from build123d import *

# Parameters (mm, degrees)
F1_DEPTH = 19.05


with BuildPart() as f1:
    # F0 (on Top) → F1 (new body)
    with BuildSketch(Plane.XY):
        with BuildLine():
            ThreePointArc((-100.25353, 101.826), (-101.667744, 101.240213), (-102.25353, 99.826))
            Line((-102.25353, 99.826), (-102.25353, -10.474))
            ThreePointArc((-102.25353, -10.474), (-101.667744, -11.888214), (-100.25353, -12.474))
            Line((-100.25353, -12.474), (-10.564581, -12.474))
            ThreePointArc((-10.564581, -12.474), (-10.036438, -12.544994), (-9.545789, -12.752936))
            Line((-9.545789, -12.752936), (77.88431, -64.507527))
            ThreePointArc((77.88431, -64.507527), (79.399684, -64.723833), (80.624166, -63.805253))
            Line((80.624166, -63.805253), (117.402527, -1.674808))
            ThreePointArc((117.402527, -1.674808), (117.618833, -0.159434), (116.700253, 1.065048))
            Line((116.700253, 1.065048), (51.127679, 39.880991))
            ThreePointArc((51.127679, 39.880991), (50.409003, 40.611496), (50.14647, 41.602056))
            Line((50.14647, 41.602056), (50.14647, 87.126))
            ThreePointArc((50.14647, 87.126), (49.560684, 88.540213), (48.14647, 89.126))
            Line((48.14647, 89.126), (-28.05353, 89.126))
            ThreePointArc((-28.05353, 89.126), (-28.549656, 89.188512), (-29.014768, 89.37214))
            Line((-29.014768, 89.37214), (-51.28878, 101.579859))
            ThreePointArc((-51.28878, 101.579859), (-51.753892, 101.763487), (-52.250017, 101.826))
            Line((-52.250017, 101.826), (-100.25353, 101.826))
        make_face()
    extrude(amount=F1_DEPTH)


solid = f1.part
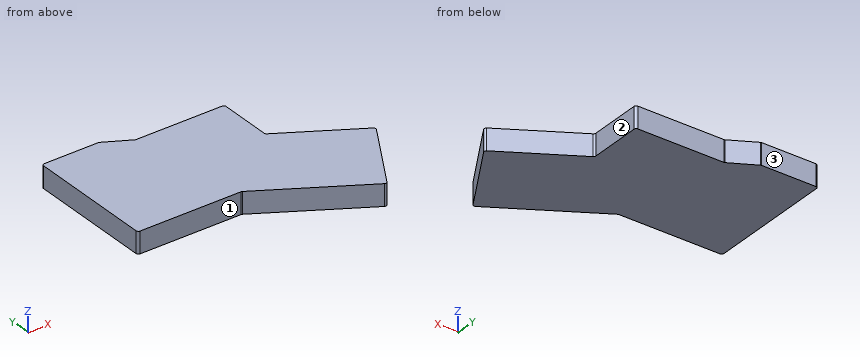
Can you work these out from the model? Positions are in its coordinate system, mm. Face numbers are marked on the shaded views. A direction names the side the tool comes from. Coordinates: 2 decimals unless noted, no trailing zeros. Write each loop counter-clockwise with the first axis right and the second up, starting at its lowest first coordinate (ties: lowest second). Pieces come first, ordered by that corner, then holes. Notation, with made-up numbers: M 17,0 L 75,0 A5 ccw 75,5 Z; hole C -28.5,22.25 d5. An arc over 180 degrees is marked long. Use one line per item in the form item = value.
Q1. I need wall thicknesses on line 1 along Y through (x, z) = (-90, 8.5); line 2 along Y through (x, z) = (-15, 10.5); line 3 along X through (y, z) = (68, 14). Which ranges of each line are inside material? Lowest first, please. Write a range as from..to.
Model answer:
line_1 = -12.47..101.83
line_2 = -12.47..89.13
line_3 = -102.25..50.15
Q2. For the marked faces 1, 2 and 3, which set-ups out of +Z, -Z, +X, -X, +Y, -Y let a thin tool reach every point of the face, with its end or its side?
Model answer:
face_1 = +Z, -Z, -X, -Y
face_2 = +Z, -Z, +X, +Y
face_3 = +Z, -Z, +X, -X, +Y
Q3. If we section it at B-B (x = -88.5): Write out the boundary of the cut face in (y, z).
Model answer:
outline = M -12.47,0 L 101.83,0 L 101.83,19.05 L -12.47,19.05 Z
Q4. If we section it at C-C (y = 73): Write out the boundary of the cut face in (x, z).
Model answer:
outline = M -102.25,0 L 50.15,0 L 50.15,19.05 L -102.25,19.05 Z
Q5. If we section it at A-A (z = 9): Write out the boundary of the cut face in (x, y).
Model answer:
outline = M -102.25,-10.47 A2 ccw -100.25,-12.47 L -10.56,-12.47 A2 cw -9.55,-12.75 L 77.88,-64.51 A2 ccw 80.62,-63.81 L 117.4,-1.67 A2 ccw 116.7,1.07 L 51.13,39.88 A2 cw 50.15,41.6 L 50.15,87.13 A2 ccw 48.15,89.13 L -28.05,89.13 A2 cw -29.01,89.37 L -51.29,101.58 A2 ccw -52.25,101.83 L -100.25,101.83 A2 ccw -102.25,99.83 Z
Q6. For P1, Ø9.5, axis at x = -44.5, z = 9, coming from the -Y side; P2, Ø6, axis at y = -48, z = 16, coming from the +X side; P3, Ø4, axis at y = -22.5, z = 7, coming from the -X side, each with a flat end and sliding along its axis, tell me the tip position at first contact or that it passes through.
Model answer:
P1 = -12.47
P2 = 91.76
P3 = 3.54
